from build123d import *

# Parameters (mm, degrees)
SKETCH1_W           = 20
SKETCH1_H           = 15
BOSS_EXTRUDE1_DEPTH = 3.5
BOSS_EXTRUDE8_DEPTH = 1.5
SKETCH3_W           = 3.4
SKETCH3_H           = 1
CUT_EXTRUDE1_DEPTH  = 18.642278764
SKETCH4_W           = 10
SKETCH4_H           = 7
BOSS_EXTRUDE9_DEPTH = 4
SKETCH5_W           = 7.5
SKETCH5_H           = 3.5
CUT_EXTRUDE2_DEPTH  = 22.592822882
CUT_EXTRUDE3_DEPTH  = 1
SKETCH7_R           = 1.25
CUT_EXTRUDE4_DEPTH  = 21.03746491


with BuildPart() as part:
    # Sketch1 → Boss-Extrude1 (new body)
    with BuildSketch(Plane.XY):
        Rectangle(SKETCH1_W, SKETCH1_H)
    extrude(amount=BOSS_EXTRUDE1_DEPTH)

    # Sketch2 → Boss-Extrude8 (add)
    with BuildSketch(Plane.XY.offset(3.5)):
        Polygon((-6.431580724, 2), (-10, 2), (-10, 1.5), (-10, 0.3), (-10, -2), (-6.431580724, -2), (-6.431580724, -1.5), (-9.8, -1.5), (-9.8, -0.2), (-6.431580724, -0.2), (-6.431580724, 0.3), (-9.8, 0.3), (-9.8, 1.5), (-6.431580724, 1.5), align=None)
        Polygon((-10, 1.5), (-10, 2), (-14, 2), (-14, -2), (-10, -2), (-10, 0.3), align=None)
    extrude(amount=BOSS_EXTRUDE8_DEPTH)

    # Sketch3 → Cut-Extrude1 (cut, through all)
    with BuildSketch(Plane.XZ.offset(2)):
        with Locations((-8.631580724, 4)):
            Rectangle(SKETCH3_W, SKETCH3_H)
    extrude(amount=-CUT_EXTRUDE1_DEPTH, mode=Mode.SUBTRACT)

    # Sketch4 → Boss-Extrude9 (add)
    with BuildSketch(Plane.XY.offset(3.5)):
        with Locations((12, 0)):
            Rectangle(SKETCH4_W, SKETCH4_H)
    extrude(amount=BOSS_EXTRUDE9_DEPTH)

    # Sketch5 → Cut-Extrude2 (cut, through all)
    with BuildSketch(Plane.XZ.offset(3.5)):
        with Locations((13.25, 5.25)):
            Rectangle(SKETCH5_W, SKETCH5_H)
    extrude(amount=-CUT_EXTRUDE2_DEPTH, mode=Mode.SUBTRACT)

    # Sketch6 → Cut-Extrude3 (cut)
    with BuildSketch(Plane.XY.offset(7.5)):
        Polygon((17, 3), (6, 3), (6, 0.25), (17, 0.25), (17, -0.25), (6, -0.25), (6, -3), (17, -3), (18, -3), (18, 3), align=None)
    extrude(amount=-CUT_EXTRUDE3_DEPTH, mode=Mode.SUBTRACT)

    # Sketch7 → Cut-Extrude4 (cut, through all)
    with BuildSketch(Plane(origin=(0, 0, 0), x_dir=(-1, 0, 0), z_dir=(0, 0, -1))):
        with Locations((8, -5)):
            Circle(SKETCH7_R)
        with Locations((8, 5)):
            Circle(SKETCH7_R)
    extrude(amount=-CUT_EXTRUDE4_DEPTH, mode=Mode.SUBTRACT)


solid = part.part
Part model, mm, in its own coordinate system. A direction names the side the tool comes from. Coordinates: 2 decimals unless noted, no trailing zeros. Order: outer loops, then holes, each group sorted by start corner. A loop starts at its lowest first (then second) coordinate and runs counter-clockwise, first axis right, second up. Notation, with made-up numbers: M 71,88.25 L 130,88.25 A13 cw 130,94.25 Z; hole C 6.5,-25.75 d3. An arc over 180 degrees is marked long. Use a Markdown table: item, result.
(1) Flat gauge pins, fed straight in: pin 1 (0.8 mm diameter, centred on x = 12.5, z = 7, fed in from -Y); pin 2 (0.8 mm diameter, centred on x = 10, z = 7, fed in from +Y); pin 3 (1.8 mm diameter, centred on y = 2.5, z = 2.5, fed in from -X); pin 4 (3 mm diameter, centred on x = 12.5, z = 5, fed in from +Y). Where does each tip first touch, or does it go through?
A:
| item | result |
|---|---|
| pin 1 | stops at y = -3.5 |
| pin 2 | stops at y = 3.5 |
| pin 3 | stops at x = -10 |
| pin 4 | passes through |
(2) Cut at C-C on y = -5.75. Write the cut outline in (x, z), then the cut area to 3 significant figures.
A:
| item | result |
|---|---|
| outline | M -10,0 L -9,0 L -9,3.5 L -10,3.5 Z; M -7,0 L 10,0 L 10,3.5 L -7,3.5 Z |
| area | 63.0 mm^2 |
(3) Tool access for faces 5 (the flat face through (11, -0.25, 7.2)), 6 (the flat face through (-10, 0, 2)), 7 (the flat face through (-11, -2, 4)), 8 (the flat face through (-10.332, 0, 4)): list every direction of +Z, -Z, +X, -X, +Y, -Y with a clear straight run to the whole face (end or side of a thin tool).
A:
| item | result |
|---|---|
| face 5 | +Z, +X, -X |
| face 6 | -Z, -X, +Y, -Y |
| face 7 | +Z, -X, -Y |
| face 8 | -Z, +Y, -Y |
(4) Cut at D-D on z = 5.5. Write the cut outline in (x, y).
A:
| item | result |
|---|---|
| outline | M 7,-3.5 L 9.5,-3.5 L 9.5,3.5 L 7,3.5 Z |
(5) Pull direction Y, two halves, no side cores. Call faces 1 (the flat face through (8, 2, 6.5)), 2 (the flat face through (0, 7.5, 2)), 3 (the flat face through (0, 0, 0)), 4 (the flat face through (9, -3.5, 6)): released by +Y, released by -Y, zero draft, split by the parting line, or undercut.
A:
| item | result |
|---|---|
| face 1 | undercut |
| face 2 | released by +Y |
| face 3 | zero draft |
| face 4 | released by -Y |
(6) Cut at B-B on x = -8. Write the cut outline in (y, z).
A:
| item | result |
|---|---|
| outline | M -7.5,0 L -6.25,0 L -6.25,3.5 L -7.5,3.5 Z; M -3.75,0 L 3.75,0 L 3.75,3.5 L -3.75,3.5 Z; M -2,4.5 L -1.5,4.5 L -1.5,5 L -2,5 Z; M -0.2,4.5 L 0.3,4.5 L 0.3,5 L -0.2,5 Z; M 1.5,4.5 L 2,4.5 L 2,5 L 1.5,5 Z; M 6.25,0 L 7.5,0 L 7.5,3.5 L 6.25,3.5 Z |
(7) Cut at A-A on y = 5. Write the cut outline in (x, z).
A:
| item | result |
|---|---|
| outline | M -10,0 L -9.25,0 L -9.25,3.5 L -10,3.5 Z; M -6.75,0 L 10,0 L 10,3.5 L -6.75,3.5 Z |
(8) Probe L1, parallel to Y at x = -8, z = 1.5; L2, parallel to Z at x = 2, y = 5.5; L3, parallel to X at y = -4, z = 2.25. List the from-to ranges inside material, lowest first.
A:
| item | result |
|---|---|
| L1 | y = -7.5 to -6.25, -3.75 to 3.75, 6.25 to 7.5 |
| L2 | z = 0 to 3.5 |
| L3 | x = -10 to -8.75, -7.25 to 10 |
